Source: CAD feature listing. Evaluate the final solid. Frame: model axes, mm. A direction names the side the tool comes from. Give positions to 0.01 mm unless a question says otherwise; leave off trailing zeros. Loops run counter-clockwise (first coordinate to the right, second up) from the corner with the lowest first, then second, coordinate; pieces in that order, holes last. Notation, with made-up numbers: (-29, 83) -> (8, 83) arc R25 cw to (8, 112) -> close; hole circle Ø8 at (4.25, 25.5). An arc over 180 degrees is marked (long way). Put each result on its own line as item: value.
```python
from build123d import *

# Parameters (mm, degrees)
SKETCH_R        = 45
PAD_DEPTH       = 8
POCKET_DEPTH    = 6
SKETCH013_R     = 2
POCKET006_DEPTH = 10
SKETCH016_W     = 35
SKETCH016_H     = 8
POCKET009_DEPTH = 5
SKETCH017_W     = 5
SKETCH017_H     = 10
POCKET010_DEPTH = 10


with BuildPart() as part:
    # Sketch → Pad (new body)
    with BuildSketch(Plane.XY):
        Circle(SKETCH_R)
    extrude(amount=PAD_DEPTH)

    # Sketch002 (on Face3 of Pad) → Pocket (cut)
    with BuildSketch(Plane.XY.offset(8)):
        Polygon((-18, 14), (-18, -14), (16.95, -14), (16.95, -12.3), (18, -11.25), (18, 6.25), (16.95, 7.3), (16.95, 14), align=None)
    extrude(amount=-POCKET_DEPTH, mode=Mode.SUBTRACT)

    # Sketch013 (on Face3 of Pocket) → Pocket006 (cut)
    with BuildSketch(Plane.XY.offset(8)):
        with Locations((-40, 0)):
            Circle(SKETCH013_R)
        with Locations((-12.363995, 38.041183)):
            Circle(SKETCH013_R)
        with Locations((32.356581, 23.51705)):
            Circle(SKETCH013_R)
        with Locations((32.366826, -23.502949)):
            Circle(SKETCH013_R)
        with Locations((-12.347418, -38.046567)):
            Circle(SKETCH013_R)
    extrude(amount=-POCKET006_DEPTH, mode=Mode.SUBTRACT)

    # Sketch016 (on Face17 of Pocket006) → Pocket009 (cut)
    with BuildSketch(Plane.XY.offset(2)):
        with Locations((-0.5, -9)):
            Rectangle(SKETCH016_W, SKETCH016_H)
        with Locations((-0.5, 9)):
            Rectangle(SKETCH016_W, SKETCH016_H)
    extrude(amount=-POCKET009_DEPTH, mode=Mode.SUBTRACT)

    # Sketch017 (on Face3 of Pocket009) → Pocket010 (cut)
    with BuildSketch(Plane.XY.offset(8)):
        with Locations((42.5, 0)):
            Rectangle(SKETCH017_W, SKETCH017_H)
    extrude(amount=-POCKET010_DEPTH, mode=Mode.SUBTRACT)


with BuildPart() as part_1:
    # Body placement: moved
    add(part.part.moved(Location((0, 0, 15))))


solid = part_1.part
```
(1) Section A-A on x = 0. Return loops of the section in (y, z), then the cut area to 3 significant figures.
Calculated:
outline: (-45, 15) -> (-13, 15) -> (-13, 17) -> (-14, 17) -> (-14, 23) -> (-45, 23) -> close; (-5, 15) -> (5, 15) -> (5, 17) -> (-5, 17) -> close; (13, 15) -> (45, 15) -> (45, 23) -> (14, 23) -> (14, 17) -> (13, 17) -> close
area: 520 mm²
(2) Section B-B on y = 0. Return loops of the section in (x, z), then the cut area to 3 significant figures.
Calculated:
outline: (-45, 15) -> (-42, 15) -> (-42, 23) -> (-45, 23) -> close; (-38, 15) -> (40, 15) -> (40, 23) -> (18, 23) -> (18, 17) -> (-18, 17) -> (-18, 23) -> (-38, 23) -> close
area: 432 mm²
(3) Reachability of faces 1 (the flat face through (0, 14, 20)), 2 (the flat face through (42, 5, 19)), 3 (the flat face through (19, 1, 23)), 4 (the flat face through (-1, -5, 16)) from +Z, -Z, +X, -X, +Y, -Y: full face, straight path, thin tool, end or side. Return the list, or none.
Calculated:
face 1: +Z
face 2: +Z, -Z, +X
face 3: +Z, +X, -X, +Y, -Y
face 4: +Z, -Z
(4) Draft query along Y for faces 5 (the flat face through (-1, 1, 15)), 6 (the flat face through (18, -3, 20)), 7 (the cylindrical face through (-44.96, 1.91, 18.94)). Return one class per face: released by +Y, released by -Y, zero draft, split by the parting line, or undercut.
Calculated:
face 5: zero draft
face 6: undercut
face 7: split by the parting line
(5) Section C-C on x = -40. Return loops of the section in (y, z), then the cut area to 3 significant figures.
Calculated:
outline: (-20.62, 15) -> (-2, 15) -> (-2, 23) -> (-20.62, 23) -> close; (2, 15) -> (20.62, 15) -> (20.62, 23) -> (2, 23) -> close
area: 298 mm²
(6) First-contact query: P1, Ø4, axis at y = -19.5, z = 17, coming from the +X side; P2, Ø0.6, axis at y = -10, z = 16, coming from the -X side; P3, Ø1, axis at x = 7, z = 16, coming from the -Y side. Flat tips, straight axial feed; report the tip coordinate or a pass-through.
Calculated:
P1: stops at x = 41.46
P2: stops at x = -43.94
P3: stops at y = -44.53
(7) Line query: probe 1 along Y at (x, z) = (32, 20.5) (3 decimals); probe 2 along Y at (x, z) = (-3, 15.5); probe 3 along Y at (x, z) = (-40, 19). Output: solid intervals per line, ascending. Write a range as from..to.
Calculated:
probe 1: y = -31.639..-25.469, -21.537..21.549, 25.485..31.639
probe 2: y = -44.9..-13, -5..5, 13..44.9
probe 3: y = -20.62..-2, 2..20.62
(8) Section D-D on z = 19.75. Return loops of the section in (x, y).
Calculated:
outline: (40, -5) -> (40, 5) -> (44.72, 5) arc R45 ccw (long way) to (44.72, -5) -> close; hole circle Ø4 at (-40, 0); hole (-18, -14) -> (16.95, -14) -> (16.95, -12.3) -> (18, -11.25) -> (18, 6.25) -> (16.95, 7.3) -> (16.95, 14) -> (-18, 14) -> close; hole circle Ø4 at (-12.36, 38.04); hole circle Ø4 at (-12.35, -38.05); hole circle Ø4 at (32.36, 23.52); hole circle Ø4 at (32.37, -23.5)
